Source: CAD feature listing. Evaluate the final solid. Frame: model axes, mm. A direction names the side the tool comes from. Coordinates: 2 decimals unless noted, no trailing zeros. Write each loop counter-clockwise with the first axis right and the second up, starting at its lowest first coordinate (ties: lowest second). Pieces come first, ordered by that corner, then holes. Notation, with made-up numbers: (6.25, 61.25) -> (51.25, 61.25) arc R17 cw to (51.25, 70.25) -> close; hole circle Ø7 at (45, 20). An arc over 180 degrees is marked (long way). One line per item, written item: value. Start each with the question number.
1. Section query A-A, the plane y = 15.5. Output: boundary loops of the cut face in (x, z), and give its area (3 significant figures).
2. Access query for faces 4 (the cylindrical face through (11.579, 47.087, 27.843)), 5 (the flat face through (0, 10, -31)), 6 (the conical face through (18.838, 63.646, -18.43)), 7 (the cylindrical face through (-8.35, 4.93, -32.89)), 8 (the flat face through (-21, 66, -22)). Directions: +Z, -Z, +X, -X, +Y, -Y. A direction counts if a zero-diameter tool reaches every point of the face in a straight line with its end or side. Return the directions, or none.
3. First-contact query: P1, Ø1.8, axis at x = 8.41, z = 31.39, coming from the +Y side; P2, Ø6, axis at x = -32, z = -7.5, coming from the +Y side; P3, Ø2.5, axis at x = 21.5, z = 21.5, coming from the +Y side; P4, Ø10, axis at y = 28.5, z = 22, coming from the +X side. Flat tips, straight axial feed; report the tip coordinate or a pass-through.
4. Mould query, pull axis X, two halves, no side actions, for faces 1 (the cylindrical face through (-20.49, 68.03, -22.61)), 2 (the flat face through (31, 10, 0)), 3 (the flat face through (0, 10, 31)). Classes: released by +X, released by -X, zero draft, split by the parting line, or undercut.
5. Line query: line 1 (X direction, y = 67.2, z = 0); line 2 (Z direction, x = -1, y = 7.5); line 3 (Y direction, x = -10, z = -11). Output: solid intervals per line, ascending.
6. Section query B-B, the plane x = -3. State how many separate pieces and enclosed holes the cut face has, and give its area (3 significant figures).
from build123d import *

# Parameters (mm, degrees)
SKETCH1_R           = 35
SKETCH1_R_2         = 30
SKETCH1_R_3         = 1.5
BOSS_EXTRUDE1_DEPTH = 65
SKETCH2_R           = 35
SKETCH2_R_2         = 1.5
SKETCH2_R_3         = 10
BOSS_EXTRUDE2_DEPTH = 5
SKETCH3_R           = 25
CUT_EXTRUDE1_DEPTH  = 60
CIRPATTERN1_COUNT   = 4
CHAMFER1_SIZE       = 5
SKETCH4_R           = 1.5
CUT_EXTRUDE2_DEPTH  = 4


with BuildPart() as part:
    # Sketch1 → Boss-Extrude1 (new body)
    with BuildSketch(Plane(origin=(0, 0, 0), x_dir=(1, 0, 0), z_dir=(0, 1, 0))):
        with Locations(Location((0, 0, 0), (0, 0, 270))):
            Circle(SKETCH1_R)
        with Locations(Location((0, 0, 0), (0, 0, 270))):
            Circle(SKETCH1_R_2, mode=Mode.SUBTRACT)
        with Locations(Location((-8.411618966, 31.392589354, 0), (0, 0, 270))):
            Circle(SKETCH1_R_3, mode=Mode.SUBTRACT)
        with Locations(Location((8.411618966, 31.392589354, 0), (0, 0, 270))):
            Circle(SKETCH1_R_3, mode=Mode.SUBTRACT)
        with Locations(Location((31.392589354, 8.411618966, 0), (0, 0, 270))):
            Circle(SKETCH1_R_3, mode=Mode.SUBTRACT)
        with Locations(Location((31.392589354, -8.411618966, 0), (0, 0, 270))):
            Circle(SKETCH1_R_3, mode=Mode.SUBTRACT)
        with Locations(Location((8.411618966, -31.392589354, 0), (0, 0, 270))):
            Circle(SKETCH1_R_3, mode=Mode.SUBTRACT)
        with Locations(Location((-8.411618966, -31.392589354, 0), (0, 0, 270))):
            Circle(SKETCH1_R_3, mode=Mode.SUBTRACT)
        with Locations(Location((-31.392589354, -8.411618966, 0), (0, 0, 270))):
            Circle(SKETCH1_R_3, mode=Mode.SUBTRACT)
        with Locations(Location((-31.392589354, 8.411618966, 0), (0, 0, 270))):
            Circle(SKETCH1_R_3, mode=Mode.SUBTRACT)
    extrude(amount=BOSS_EXTRUDE1_DEPTH)

    # Sketch2 → Boss-Extrude2 (add)
    with BuildSketch(Plane(origin=(0, 65, 0), x_dir=(1, 0, 0), z_dir=(0, 1, 0))):
        with Locations(Location((0, 0, 0), (0, 0, 270))):
            Circle(SKETCH2_R)
        with Locations(Location((-8.411618966, 31.392589354, 0), (0, 0, 270))):
            Circle(SKETCH2_R_2, mode=Mode.SUBTRACT)
        with Locations(Location((8.411618966, 31.392589354, 0), (0, 0, 270))):
            Circle(SKETCH2_R_2, mode=Mode.SUBTRACT)
        with Locations(Location((31.392589354, 8.411618966, 0), (0, 0, 270))):
            Circle(SKETCH2_R_2, mode=Mode.SUBTRACT)
        with Locations(Location((31.392589354, -8.411618966, 0), (0, 0, 270))):
            Circle(SKETCH2_R_2, mode=Mode.SUBTRACT)
        with Locations(Location((8.411618966, -31.392589354, 0), (0, 0, 270))):
            Circle(SKETCH2_R_2, mode=Mode.SUBTRACT)
        with Locations(Location((-8.411618966, -31.392589354, 0), (0, 0, 270))):
            Circle(SKETCH2_R_2, mode=Mode.SUBTRACT)
        with Locations(Location((-31.392589354, -8.411618966, 0), (0, 0, 270))):
            Circle(SKETCH2_R_2, mode=Mode.SUBTRACT)
        with Locations(Location((-31.392589354, 8.411618966, 0), (0, 0, 270))):
            Circle(SKETCH2_R_2, mode=Mode.SUBTRACT)
        with Locations(Location((0, 0, 0), (0, 0, 270))):
            Circle(SKETCH2_R_3, mode=Mode.SUBTRACT)
    extrude(amount=BOSS_EXTRUDE2_DEPTH)

    # Sketch3 → Cut-Extrude1 (cut)
    with BuildSketch(Plane(origin=(0, 70, 0), x_dir=(1, 0, 0), z_dir=(0, 1, 0))):
        with Locations((0, 50)):
            Circle(SKETCH3_R)
    cut_extrude1 = extrude(amount=-CUT_EXTRUDE1_DEPTH, mode=Mode.SUBTRACT)

    # CirPattern1: Cut-Extrude1 ×4 about axis
    cirpattern1_axis = Axis((0, 0, 0), (0, 1, 0))
    for i in range(1, CIRPATTERN1_COUNT):
        add(cut_extrude1.rotate(cirpattern1_axis, i * 360 / CIRPATTERN1_COUNT), mode=Mode.SUBTRACT)

    # Chamfer1
    chamfer1_edges = [part.edges().sort_by_distance(p)[0] for p in [
        (-21.213203436, 65, -21.213203436),
        (21.213203436, 65, 21.213203436),
        (21.213203436, 65, -21.213203436),
        (-21.213203436, 65, 21.213203436),
    ]]
    chamfer(chamfer1_edges, length=CHAMFER1_SIZE - 0.0001)  # a hair under: the kernel refuses the full size

    # Sketch4 → Cut-Extrude2 (cut)
    with BuildSketch(Plane(origin=(0, 70, 0), x_dir=(1, 0, 0), z_dir=(0, 1, 0))):
        with Locations(Location((-21.5, 21.5, 0), (0, 0, 270))):
            Circle(SKETCH4_R)
        with Locations(Location((21.5, 21.5, 0), (0, 0, 270))):
            Circle(SKETCH4_R)
        with Locations(Location((21.5, -21.5, 0), (0, 0, 270))):
            Circle(SKETCH4_R)
        with Locations(Location((-21.5, -21.5, 0), (0, 0, 270))):
            Circle(SKETCH4_R)
    extrude(amount=-CUT_EXTRUDE2_DEPTH, mode=Mode.SUBTRACT)


solid = part.part
Computed values:
1. outline: (-31, -16.25) arc R35 ccw to (-16.25, -31) arc R25 cw to (-11.4, -27.75) arc R30 cw to (-27.75, -11.4) arc R25 cw to start; (-31, 16.25) arc R25 cw to (-27.75, 11.4) arc R30 cw to (-11.4, 27.75) arc R25 cw to (-16.25, 31) arc R35 ccw to start; (11.4, -27.75) arc R25 cw to (16.25, -31) arc R35 ccw to (31, -16.25) arc R25 cw to (27.75, -11.4) arc R30 cw to start; (11.4, 27.75) arc R30 cw to (27.75, 11.4) arc R25 cw to (31, 16.25) arc R35 ccw to (16.25, 31) arc R25 cw to start
1. area: 443 mm²
2. face 4: +Z, +Y
2. face 5: -Z, +Y
2. face 6: -Y
2. face 7: +Y, -Y
2. face 8: +Y
3. P1: passes through
3. P2: stops at y = 10
3. P3: stops at y = 66
3. P4: stops at x = 30.59
4. face 1: undercut
4. face 2: zero draft
4. face 3: undercut
5. line 1: x = -25 to -10, 10 to 25
5. line 2: z = -34.99 to -29.98, 29.98 to 34.99
5. line 3: y = 65 to 70
6. separate pieces: 4
6. enclosed holes: 0
6. area: 257 mm²
